Model file for the job. Use its own axes, mm. A direction names the side the tool comes from. Round coordinates to 2 decimals unless told otherwise and drop trailing zeros. Write each loop counter-clockwise with the first axis right and the second up, starting at its lowest first coordinate (ties: lowest second). Pieces come first, ordered by that corner, then holes. Notation, with made-up numbers: (36.5, -0.5) - (42.5, -0.5) arc R27 ccw to (42.5, 37.5) - close; hole circle Ø1 at (-35.75, -24). An arc over 180 degrees is marked (long way). One line per item, written item: value.
from build123d import *

# Parameters (mm, degrees)
SKETCH_2_R               = 1.25
CUT_EXTRUDE_1_DEPTH      = 8
PATTERN_CIRCULAR_1_COUNT = 8
SKETCH_3_R               = 1.55
CUT_EXTRUDE_2_DEPTH      = 41.137264585


with BuildPart() as part:
    # 草图1 → 旋转1 (revolve)
    with BuildSketch(Plane.XY, mode=Mode.PRIVATE) as revolve_1_sk:
        Polygon((-16, 0), (-17, 0), (-17, 2), (-21, 2), (-21, 6), (-17.5, 8.020725942), (-17.5, 27), (-6.75, 27), (-6.75, 25), (-16, 25), align=None)
    revolve(revolve_1_sk.sketch.rotate(Axis((0, 0, 0), (0, 1, 0)), 270), axis=Axis((0, 0, 0), (0, 1, 0)))

    # 草图2 → 切除-拉伸1 (cut)
    with BuildSketch(Plane.XZ.offset(-2)):
        with Locations(Location((0, -19, 0), (0, 0, 270))):
            Circle(SKETCH_2_R)
    cut_extrude_1 = extrude(amount=-CUT_EXTRUDE_1_DEPTH, mode=Mode.SUBTRACT)

    # 阵列(圆周)1: 切除-拉伸1 ×8 about axis
    pattern_circular_1_axis = Axis((0, 0, 0), (0, 1, 0))
    for i in range(1, PATTERN_CIRCULAR_1_COUNT):
        add(cut_extrude_1.rotate(pattern_circular_1_axis, i * 360 / PATTERN_CIRCULAR_1_COUNT), mode=Mode.SUBTRACT)

    # 草图3 → 切除-拉伸2 (cut, through all)
    with BuildSketch(Plane(origin=(0, 27, 0), x_dir=(1, 0, 0), z_dir=(0, 1, 0))):
        with Locations(Location((0, -9.5, 0), (0, 0, 270))):
            Circle(SKETCH_3_R)
        with Locations(Location((-8.227241336, 4.75, 0), (0, 0, 270))):
            Circle(SKETCH_3_R)
        with Locations(Location((8.227241336, 4.75, 0), (0, 0, 270))):
            Circle(SKETCH_3_R)
    extrude(amount=-CUT_EXTRUDE_2_DEPTH, mode=Mode.SUBTRACT)


solid = part.part
1. Mould opens along Z. For faces 3 (the face through (-6.31, 4.03, -20.03)), 4 (the face through (10, 0, 13)), 5 (the face through (15.62, 12.32, 3.47)) say: released by +Z, released by -Z, zero draft, split by the parting line, or undercut.
Report:
face 3: split by the parting line
face 4: zero draft
face 5: undercut
2. Band-saw the part on C-C on y = 17.5. Write the cut outline in (x, z), plus the area to 3 significant figures.
Report:
outline: circle Ø35 at (0, 0); hole circle Ø32 at (0, 0)
area: 158 mm²
3. Drop flat-ended pins along their axis: pin 1 (4 mm diameter, centred on x = 0, z = 9.5, fed in from -Y); pin 2 (3 mm diameter, centred on x = 3, y = 5.5, fed in from +Z); pin 3 (1.5 mm diameter, centred on y = 13, z = 6, fed in from -X). Give the stop position or say it passes through.
Report:
pin 1: y = 25
pin 2: z = 20.95
pin 3: x = -16.69
4. Band-saw the part on B-B on x = 0. State how many separate pieces and enclosed holes the cut face has, plus the area to 3 significant figures.
Report:
separate pieces: 5
enclosed holes: 0
area: 119 mm²
5. Wall check: probe 1 along Z at (x, y) = (12.5, 5.25); probe 2 along Y at (x, z) = (-9.5, -3); probe 3 along Z at (x, y) = (-13, 18). Give the ranges that are in metal, low to high. Write a range as [from, to].
Report:
probe 1: [-16.87, -14.26], [-12.61, -9.99], [9.99, 12.61], [14.26, 16.87]
probe 2: [25, 27]
probe 3: [-11.72, -9.33], [9.33, 11.72]
6. Tool access for faces 1 (the face through (0.05, 4.24, -17.75)), 2 (the face through (-17.2, 2, -0.1)): list every direction of +Z, -Z, +X, -X, +Y, -Y with a clear straight run to the whole face (end or side of a thin tool).
Report:
face 1: +Y, -Y
face 2: -Y
7. Band-saw the part on A-A on z = 0. Write the cut outline in (x, y).
Report:
outline: (-21, 2) - (-20.25, 2) - (-20.25, 6.43) - (-21, 6) - close; (-17.75, 2) - (-17, 2) - (-17, 0) - (-16, 0) - (-16, 25) - (-6.75, 25) - (-6.75, 27) - (-17.5, 27) - (-17.5, 8.02) - (-17.75, 7.88) - close; (6.75, 25) - (16, 25) - (16, 0) - (17, 0) - (17, 2) - (17.75, 2) - (17.75, 7.88) - (17.5, 8.02) - (17.5, 27) - (6.75, 27) - close; (20.25, 2) - (21, 2) - (21, 6) - (20.25, 6.43) - close
